Design review of the part built by this model. Coordinates are the model's own, in mm. Face numbers are marked on the shaded views. A direction names the side the tool comes from. Coordinates: 2 decimals unless noted, no trailing zeros. Loops run counter-clockwise (first coordinate to the right, second up) from the corner with the lowest first, then second, coordinate; pieces in that order, holes last. Notation, with made-up numbers: (11, 4) -> (38, 4) arc R12 ccw to (38, 11) -> close; hole circle Ø9 at (-30, -15). An arc over 180 degrees is marked (long way). Use a Markdown table: item, result. Add a question column.
Q1. Take a section at D-D on y = 3.5. Write out the cut boundary in (x, z) (3 decimals), plus the area to 3 significant figures.
Q2. Take a section at C-C on y = 9.5. Write out the cut boundary in (x, z).
Q3. Take a section at A-A on x = 15. Write out the cut boundary in (y, z) (3 decimals).
Q4. For probe 1 along Y at (x, z) = (1.5, 10); probe 2 along Z at (x, y) = (15, 2.2) (3 decimals), list the stretches that pass through material, from the lowest coordinate up.
Q5. For the marked faces 1 and 2, list the 3-axis set-ups (+Z, -Z, +X, -X, +Y, -Y) from which the entire face can be reached by the end or side of a thin tool; tool diameter is ignored.
Q6. Take a section at B-B on z = 10. Write out the cut boundary in (x, y) (3 decimals), plus the area to 3 significant figures.
Q7. Draft analysis for pull direction Z (two halves, no side actions). For the marked faces 3, 4, 5 and 6, state which applies: pulls with the +Z half, pulls with the -Z half, needs draft (parallel to the pull), parting line crosses it, or undercut.
Q8. Clearance check with flat-ended pins moving along their axes: pin 1 Ø6 at (x, z) = (27, 11.5) entering from +Y; pin 2 Ø10 at (y, z) = (15.5, 10.5) entering from +X. State where each tip first meets the part, or that it passes through.
from build123d import *

# Parameters (mm, degrees)
BOSS_EXTRUDE1_DEPTH = 20
SKETCH2_R           = 1.755
CUT_EXTRUDE1_DEPTH  = 20
SKETCH3_R           = 2.5
CUT_EXTRUDE2_DEPTH  = 20


with BuildPart() as part:
    # Sketch1 → Boss-Extrude1 (new body)
    with BuildSketch(Plane.XY):
        with BuildLine():
            Line((0, 20), (0, 0))
            Line((0, 0), (30, 0))
            Line((30, 0), (30, 5.78313253))
            Line((30, 5.78313253), (10, 5.78313253))
            ThreePointArc((10, 5.78313253), (6.464466094, 7.247598624), (5, 10.78313253))
            Line((5, 10.78313253), (5, 20))
            Line((5, 20), (0, 20))
        make_face()
    extrude(amount=BOSS_EXTRUDE1_DEPTH)

    # Sketch2 → Cut-Extrude1 (cut)
    with BuildSketch(Plane.XZ):
        with Locations((15, 10)):
            Circle(SKETCH2_R)
    extrude(amount=-CUT_EXTRUDE1_DEPTH, mode=Mode.SUBTRACT)

    # Sketch3 → Cut-Extrude2 (cut)
    with BuildSketch(Plane.ZY):
        with Locations((10, 10)):
            Circle(SKETCH3_R)
    extrude(amount=-CUT_EXTRUDE2_DEPTH, mode=Mode.SUBTRACT)


solid = part.part
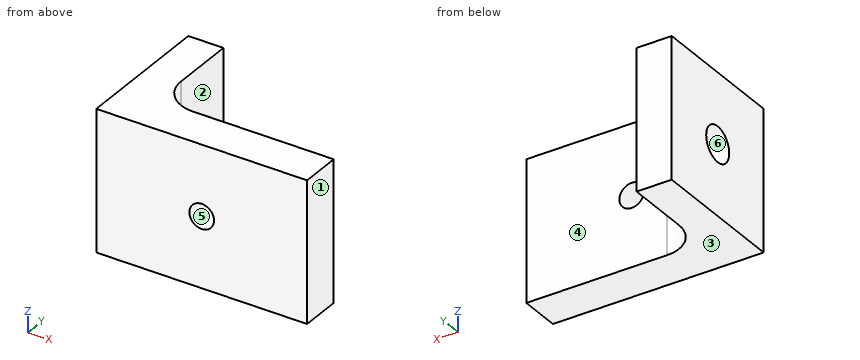
Answer list:
| question | item | result |
|---|---|---|
| 1 | outline | (0, 0) -> (30, 0) -> (30, 20) -> (0, 20) -> close; hole circle Ø3.51 at (15, 10) |
| 1 | area | 590 mm² |
| 2 | outline | (0, 0) -> (5.17, 0) -> (5.17, 7.55) -> (0, 7.55) -> close; (0, 12.45) -> (5.17, 12.45) -> (5.17, 20) -> (0, 20) -> close |
| 3 | outline | (0, 0) -> (5.783, 0) -> (5.783, 8.245) -> (0, 8.245) -> close; (0, 11.755) -> (5.783, 11.755) -> (5.783, 20) -> (0, 20) -> close |
| 4 | probe 1 | 0 to 7.5, 12.5 to 20 |
| 4 | probe 2 | 0 to 8.245, 11.755 to 20 |
| 5 | face 1 | +Z, -Z, +X, +Y, -Y |
| 5 | face 2 | +Z, -Z, +X, +Y |
| 6 | outline | (0, 0) -> (13.245, 0) -> (13.245, 5.783) -> (10, 5.783) arc R5 cw to (6.229, 7.5) -> (0, 7.5) -> close; (0, 12.5) -> (5, 12.5) -> (5, 20) -> (0, 20) -> close; (16.755, 0) -> (30, 0) -> (30, 5.783) -> (16.755, 5.783) -> close |
| 6 | area | 203 mm² |
| 7 | face 3 | pulls with the -Z half |
| 7 | face 4 | needs draft |
| 7 | face 5 | undercut |
| 7 | face 6 | undercut |
| 8 | pin 1 | y = 5.78 |
| 8 | pin 2 | x = 5 |
